Can you work these out from the model? Positions are in its coordinate system, mm. A direction names the side the tool comes from. Round coordinates to 2 decimals unless told otherwise and drop trailing zeros. Loops run counter-clockwise (first coordinate to the right, second up) from the corner with the lowest first, then second, coordinate; pieces in that order, holes last.
from build123d import *

# Parameters (mm, degrees)
SKETCH1_W                = 10
SKETCH1_H                = 1.6
BOSS_EXTRUDE1_DEPTH      = 15
BOSS_EXTRUDE1_TAPER      = -7
SHELL1_T                 = -0.5
SKETCH6_W                = 3.4
SKETCH6_H                = 20
BOSS_EXTRUDE2_DEPTH      = 3.5
BOSS_EXTRUDE2_2_DEPTH    = 3.5
CUT_EXTRUDE11_DEPTH      = 10
CUT_EXTRUDE11_DEPTH_BACK = 10
SKETCH11_RX              = 4.5
SKETCH11_RY              = 1.5
CUT_EXTRUDE12_DEPTH      = 10
BOSS_EXTRUDE3_DEPTH      = 0.5
SKETCH20_R               = 1.499118307
BOSS_EXTRUDE4_DEPTH      = 2.5
SKETCH22_R               = 1.001403974
CUT_EXTRUDE13_DEPTH      = 13
SKETCH25_W               = 2
SKETCH25_H               = 1.4
CUT_EXTRUDE14_DEPTH      = 1.5
SKETCH28_R               = 1.498355692
BOSS_EXTRUDE5_DEPTH      = 2.5
SKETCH29_R               = 1.002174376
CUT_EXTRUDE15_DEPTH      = 13
SKETCH30_W               = 3.2
SKETCH30_H               = 1.6
BOSS_EXTRUDE6_DEPTH      = 9
BOSS_EXTRUDE6_TAPER      = -6


with BuildPart() as part:
    # Sketch1 → Boss-Extrude1 (new body)
    with BuildSketch(Plane(origin=(0, 0, 0), x_dir=(1, 0, 0), z_dir=(0, 1, 0))):
        Rectangle(SKETCH1_W, SKETCH1_H)
    extrude(amount=BOSS_EXTRUDE1_DEPTH, taper=BOSS_EXTRUDE1_TAPER)

    # Shell1
    shell1_openings = [part.faces().sort_by_distance(p)[0] for p in [
        (0, 15, 0),
    ]]
    offset(amount=SHELL1_T, openings=shell1_openings, kind=Kind.INTERSECTION)

    # Sketch11 → Cut-Extrude11 (cut, two sides: drawn at the far end of the back side and taken through both)
    with BuildSketch(Plane.XY.offset(-CUT_EXTRUDE11_DEPTH_BACK)):
        with Locations((0, 15)):
            Ellipse(SKETCH11_RX, SKETCH11_RY)
    extrude(amount=CUT_EXTRUDE11_DEPTH + CUT_EXTRUDE11_DEPTH_BACK, mode=Mode.SUBTRACT)

    # Sketch18 → Cut-Extrude12 (cut, symmetric)
    with BuildSketch(Plane.XY):
        Polygon((-2.966549011, 13.872092056), (-6.188554642, 9.680000756), (-6.937287507, 15.777940591), (-2.966549011, 15.777940591), align=None)
    cut_extrude12 = extrude(amount=CUT_EXTRUDE12_DEPTH, both=True, mode=Mode.SUBTRACT)

    # Sketch19 → Boss-Extrude3 (add)
    with BuildSketch(Plane(origin=(-8.567447802, 6.584867333, 0), x_dir=(0, 0, 1), z_dir=(-0.7928688844776028, 0.6093922644957365, 0))):
        Polygon((1.988554642, 3.903714074), (2.503278732, 9.190958134), (-2.503278732, 9.190958134), (-1.988554642, 3.903714074), align=None)
    boss_extrude3 = extrude(amount=-BOSS_EXTRUDE3_DEPTH)

    # Mirror2: Cut-Extrude12 across plane
    add(cut_extrude12.mirror(Plane(origin=(0, 0, 0), x_dir=(0, 0, 1), z_dir=(1, 0, 0))), mode=Mode.SUBTRACT)

    # Mirror3: Boss-Extrude3 across plane
    add(boss_extrude3.mirror(Plane(origin=(0, 0, 0), x_dir=(0, 0, 1), z_dir=(1, 0, 0))))


with BuildPart() as body_2:
    # Sketch6 → Boss-Extrude2 (new body)
    with BuildSketch(Plane.XZ):
        with Locations((-3.3, 0)):
            Rectangle(SKETCH6_W, SKETCH6_H)
    extrude(amount=-BOSS_EXTRUDE2_DEPTH)


with BuildPart() as body_3:
    # Sketch6 → Boss-Extrude2 2 (new body)
    with BuildSketch(Plane.XZ):
        with Locations((3.3, 0)):
            Rectangle(SKETCH6_W, SKETCH6_H)
    extrude(amount=-BOSS_EXTRUDE2_2_DEPTH)

    # Sketch20 → Boss-Extrude4 (add)
    with BuildSketch(Plane.XY.offset(10)):
        with Locations((3.3, 1.75)):
            Circle(SKETCH20_R)
    extrude(amount=BOSS_EXTRUDE4_DEPTH)


with BuildPart() as cut_extrude13_tool:
    # Sketch22 → Cut-Extrude13 (new body)
    with BuildSketch(Plane.XY.offset(12.5)):
        with Locations((3.3, 1.75)):
            Circle(SKETCH22_R)
    extrude(amount=-CUT_EXTRUDE13_DEPTH)


with BuildPart() as part_1:
    add(part.part)

    # Cut-Extrude13: cut by cut_extrude13_tool
    add(cut_extrude13_tool.part, mode=Mode.SUBTRACT)


with BuildPart() as body_3_1:
    add(body_3.part)

    # Cut-Extrude13: cut by cut_extrude13_tool
    add(cut_extrude13_tool.part, mode=Mode.SUBTRACT)


with BuildPart() as cut_extrude14_tool:
    # Sketch25 → Cut-Extrude14 (new body)
    with BuildSketch(Plane(origin=(0, 3.5, 0), x_dir=(1, 0, 0), z_dir=(0, 1, 0))):
        with Locations((-3.371950412, 0.026080252)):
            Rectangle(SKETCH25_W, SKETCH25_H)
    cut_extrude14 = extrude(amount=-CUT_EXTRUDE14_DEPTH)


with BuildPart() as part_2:
    add(part_1.part)

    # Cut-Extrude14: cut by cut_extrude14_tool
    add(cut_extrude14_tool.part, mode=Mode.SUBTRACT)


with BuildPart() as body_2_1:
    add(body_2.part)

    # Cut-Extrude14: cut by cut_extrude14_tool
    add(cut_extrude14_tool.part, mode=Mode.SUBTRACT)

    # Sketch28 → Boss-Extrude5 (add)
    with BuildSketch(Plane.XY.offset(10)):
        with Locations((-3.3, 1.75)):
            Circle(SKETCH28_R)
    extrude(amount=BOSS_EXTRUDE5_DEPTH)


with BuildPart() as mirror6_tool:
    # Mirror6: Cut-Extrude14 across plane
    add(cut_extrude14.mirror(Plane(origin=(0, 0, 0), x_dir=(0, 0, 1), z_dir=(1, 0, 0))))


with BuildPart() as part_3:
    add(part_2.part)

    # Mirror6: cut by mirror6_tool
    add(mirror6_tool.part, mode=Mode.SUBTRACT)


with BuildPart() as body_3_2:
    add(body_3_1.part)

    # Mirror6: cut by mirror6_tool
    add(mirror6_tool.part, mode=Mode.SUBTRACT)


with BuildPart() as cut_extrude15_tool:
    # Sketch29 → Cut-Extrude15 (new body)
    with BuildSketch(Plane.XY.offset(12.5)):
        with Locations((-3.3, 1.75)):
            Circle(SKETCH29_R)
    extrude(amount=-CUT_EXTRUDE15_DEPTH)


with BuildPart() as part_4:
    add(part_3.part)

    # Cut-Extrude15: cut by cut_extrude15_tool
    add(cut_extrude15_tool.part, mode=Mode.SUBTRACT)



with BuildPart() as body_2_2:
    add(body_2_1.part)

    # Cut-Extrude15: cut by cut_extrude15_tool
    add(cut_extrude15_tool.part, mode=Mode.SUBTRACT)


with BuildPart() as part_5:
    add(part_4.part)

    add(body_2_2.part)  # Boss-Extrude6 merges body 2

    add(body_3_2.part)  # Boss-Extrude6 merges body 3
    # Sketch30 → Boss-Extrude6 (add)
    with BuildSketch(Plane.XZ):
        Rectangle(SKETCH30_W, SKETCH30_H)
    extrude(amount=-BOSS_EXTRUDE6_DEPTH, taper=BOSS_EXTRUDE6_TAPER)


solid = part_5.part
(1) For faces 1 (the flat face through (-1.6, 2, -5)), 2 (the flat face through (1.6, 2, 5)), 3 (the flat face through (-4.372, 3, 0)), 4 (the cylindrical face through (-1.87, 2.2, 11.23)), which set-ups out of +Z, -Z, +X, -X, +Y, -Y let a thin tool reach every point of the face, with its end or its side?
Worked answers:
face 1: -Z, -Y
face 2: +Z, -Y
face 3: none
face 4: +Z
(2) If we section it at B-B, the plane y = 4: State how many separate pieces and enclosed holes the cut face has, then the cut area to 3 significant figures.
Worked answers:
separate pieces: 1
enclosed holes: 2
area: 19.0 mm2
(3) If we section it at A-A, the plane z = -3.5: List the corners of the cut face in (x, y) for me, then the cut area to 3 significant figures.
Worked answers:
outline: (-5, 0) - (-1.6, 0) - (-1.6, 3.5) - (-5, 3.5) - close; (1.6, 0) - (5, 0) - (5, 3.5) - (1.6, 3.5) - close
area: 23.8 mm2
(4) Will these pins go through, and if not, where does the flat tip stop? P1, Ø1.5, axis at y = 3, z = -0.5, coming from the +X side; P2, Ø1.1, axis at y = 1, z = 6.5, coming from the +X side; P3, Ø1.6, axis at x = 3, z = -0.5, coming from the +Y side; P4, Ø5, axis at x = 0.5, y = 8.5, coming from the -Z side.
Worked answers:
P1: stops at x = 5.46
P2: stops at x = 5
P3: stops at y = 13.87
P4: stops at z = -2.15
(5) If we mould it in two halves opening along Z, with no side actions, what happens to faces 5 (the flat face through (3, 3.5, 6)), 6 (the flat face through (3, 1, -0.5)), 7 (the flat face through (-5.384, 7.232, -0.021))? For each: released by +Z, released by -Z, zero draft, split by the parting line, or undercut.
Worked answers:
face 5: zero draft
face 6: released by +Z
face 7: undercut
(6) If I drill on line 1 (X direction, y = 1.75, z = 3.25); line 2 (X direction, y = 1, z = -8); line 3 (Y direction, x = 3.3, z = 4), over which ranges is the centre line in solid material (lowest first)?
Worked answers:
line 1: x = -5 to -4.3, -2.3 to -1.6, 1.6 to 2.3, 4.3 to 5
line 2: x = -5 to -1.6, 1.6 to 5
line 3: y = 0 to 0.75, 2.75 to 3.5
